Could you check a few things on this drawing? It's one solid part, dimensions in mm from its lowest x, y, z. A direction names the side the tool comes from. Give positions to 0.01 mm unless a question says otherwise; leave off trailing zeros. Loops run counter-clockwise (first coordinate to the right, second up) from the corner with the lowest first, then second, coordinate; pieces in that order, holes last. Notation, with made-up numbers: (-30, -17.75) - (-7, -17.75) arc R35 cw to (-7, 20.25) - close; hole circle Ø3 at (-30.75, -30.5). An arc over 180 degrees is marked (long way). Use CSV: the item, a comma, the result in double quotes.
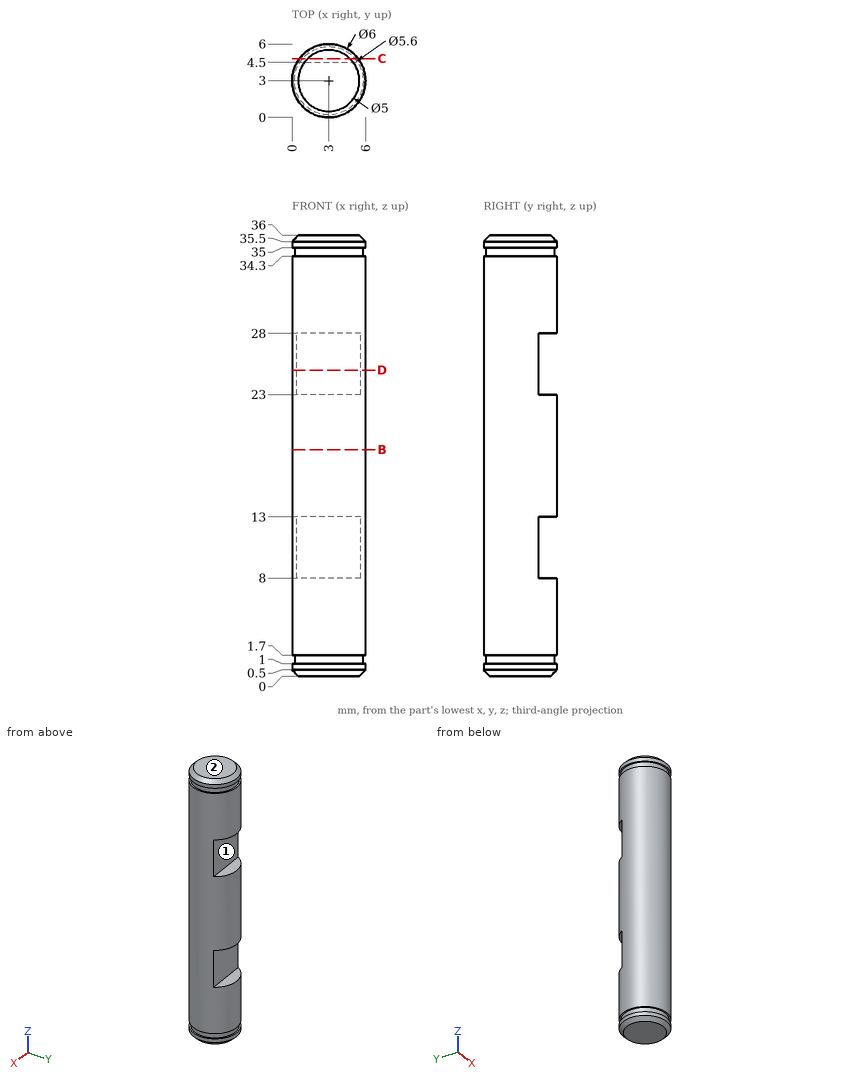
1) Suppose I cut it at C-C (y = 4.8). State how many separate pieces and enclosed holes the cut face has, plus the area to 3 significant figures.
Answer below:
separate pieces,"3"
enclosed holes,"0"
area,"123 mm2"
2) I need wall thicknesses on line 1 along Z through (x, y) = (2.2, 4.95); line 2 along Z through (x, y) = (0.7, 2); line 3 along Y through (x, z) = (1.5, 7). Which ranges of each line are inside material? Lowest first, please.
Answer below:
line 1,"z = 0 to 8, 13 to 23, 28 to 36"
line 2,"z = 0.01 to 35.99"
line 3,"y = 0.4 to 5.6"
3) Suppose I cut it at D-D (z = 25). Please give me the cut outline in (x, y), plus the area to 3 significant figures.
Answer below:
outline,"(0.4, 4.5) arc R3 ccw (long way) to (5.6, 4.5) - close"
area,"22.7 mm2"
4) Suppose I cut it at B-B (z = 18.5). Please give me the cut outline in (x, y), plus the area to 3 significant figures.
Answer below:
outline,"circle Ø6 at (3, 3)"
area,"28.3 mm2"
5) I'm going to push flat-ended pins straight in: P1, Ø3, axis at y = 1.5, z = 25, coming from the +X side; P2, Ø1.5, axis at y = 2, z = 16.5, coming from the -X side; P3, Ø2.5, axis at x = 2, z = 11.5, coming from the +Y side. Where does each tip first touch, or does it pass through?
Answer below:
P1,"stops at x = 6"
P2,"stops at x = 0.01"
P3,"stops at y = 4.5"
6) Which directions (+Z, -Z, +X, -X, +Y, -Y) give clear straight access to the entire face, cutting with the end or side of a thin tool? Please do the marked faces 1 and 2.
Answer below:
face 1,"+X, -X, +Y"
face 2,"+Z, +X, -X, +Y, -Y"
